Geometry: final body of the model. Coordinates: model frame, mm. Give positions to 0.01 mm unless a question says otherwise; leave off trailing zeros. Loops run counter-clockwise (first coordinate to the right, second up) from the corner with the lowest first, then second, coordinate; pieces in that order, holes last.
from build123d import *

# Parameters (mm, degrees)
SKETCH1_W           = 190.5
SKETCH1_H           = 57.15
BOSS_EXTRUDE1_DEPTH = 6.35
SKETCH3_R           = 3.175
CUT_EXTRUDE2_DEPTH  = 7.35


with BuildPart() as part:
    # Sketch1 → Boss-Extrude1 (new body)
    with BuildSketch(Plane(origin=(0, 0, 0), x_dir=(1, 0, 0), z_dir=(0, 1, 0))):
        Rectangle(SKETCH1_W, SKETCH1_H)
    extrude(amount=BOSS_EXTRUDE1_DEPTH)

    # Sketch3 → Cut-Extrude2 (cut, through all)
    with BuildSketch(Plane.XZ):
        with Locations((-80.645, -19.05)):
            Circle(SKETCH3_R)
        with Locations((-39.243, 19.05)):
            Circle(SKETCH3_R)
    cut_extrude2 = extrude(amount=-CUT_EXTRUDE2_DEPTH, mode=Mode.SUBTRACT)

    # Mirror1: Cut-Extrude2 across plane
    add(cut_extrude2.mirror(Plane(origin=(0, 0, 0), x_dir=(0, 0, 1), z_dir=(1, 0, 0))), mode=Mode.SUBTRACT)


solid = part.part
Item 1: Ray query, probe 1 along X at (y, z) = (2.5, 19.5); probe 2 along X at (y, z) = (4.5, 18); probe 3 along Z at (x, y) = (-38.5, 5.75) (3 decimals). Return the intervals inside material, ascending.
Values follow:
probe 1: x = -95.25 to -42.39, -36.1 to 36.1, 42.39 to 95.25
probe 2: x = -95.25 to -42.24, -36.25 to 36.25, 42.24 to 95.25
probe 3: z = -28.575 to 15.963, 22.137 to 28.575
Item 2: Section query A-A on z = -19.05. Return loops of the section in (x, y).
Values follow:
outline: (-95.25, 0) - (-83.82, 0) - (-83.82, 6.35) - (-95.25, 6.35) - close; (-77.47, 0) - (77.47, 0) - (77.47, 6.35) - (-77.47, 6.35) - close; (83.82, 0) - (95.25, 0) - (95.25, 6.35) - (83.82, 6.35) - close
Item 3: Draft query along X for faces 1 (the face through (83.817, 3.131, -18.91)), 2 (the face through (95.25, 3, 0)), 3 (the face through (-1, 0, 0)). Return one class per face: +X half, -X half, draft (parallel to the pull), parting line (faces both ways), or undercut.
Values follow:
face 1: undercut
face 2: +X half
face 3: draft
